Verification items for the finished model (mm, model axes). A direction names the side the tool comes from. Coordinates: 2 decimals unless noted, no trailing zeros. Order: outer loops, then holes, each group sorted by start corner. A loop starts at its lowest first (then second) coordinate and runs counter-clockwise, first axis right, second up. Notation, with made-up numbers: (4, -9.5) -> (26, -9.5) arc R26 cw to (26, 15.5) -> close; hole circle Ø4 at (82.25, -29). An arc over 180 degrees is marked (long way). Use CSV: the item, a comma, the result in double quotes. Start each with the question number.
1) Go/stop test with a flat-tipped pin: pin 1 (2.5 mm diameter, centred on x = -6, z = -2, fed in from +Y). Record where the tip stops, or that it passes through.
2) Scan lines: line 1 along Y through (x, z) = (-5.65, 1.25); line 2 along Z through (x, y) = (-5.75, -19.75); line 3 along Y through (x, z) = (-4.25, -2.3). Record each from-to range of solid material in increasing order.
3) Sectioned sample at C-C on x = -9. Record the boundary of the cut face in (y, z), then the cut area to 3 significant figures.
4) Sectioned sample at D-D on z = 0.35. Record the boundary of the cut face in (x, y).
5) Sectioned sample at B-B on y = -14. Record the boundary of the cut face in (x, z), then the cut area to 3 significant figures.
6) Release check for a two-part mould opening along Y. For faces 1 (the flat face through (-6, -11, 0)), 2 (the flat face through (-6, -23, 0)), 3 (the cylindrical face through (-4.76, -13.44, 1.48)) record: released by +Y, released by -Y, zero draft, split by the parting line, or undercut.
7) Sectioned sample at A-A on x = -5.65. Record the boundary of the cut face in (y, z), then the cut area to 3 significant figures.
8) Tool access check on faces 4 (the flat face through (-6, -13, 3)), 5 (the flat face through (-6, -20, -1)). Record the directions out of +Z, -Z, +X, -X, +Y, -Y that give a thin tool (end or side, any length) a straight path to the whole face; none if there is none.
from build123d import *

# Parameters (mm, degrees)
SKETCH1_W           = 7.7
SKETCH1_H           = 17
SKETCH1_R           = 1.65
BOSS_EXTRUDE1_DEPTH = 3
SKETCH2_W           = 7.7
SKETCH2_H           = 6
BOSS_EXTRUDE2_DEPTH = 3


with BuildPart() as part:
    # Sketch1 → Boss-Extrude1 (new body)
    with BuildSketch(Plane.XY):
        with Locations((-5.65, -11.5)):
            Rectangle(SKETCH1_W, SKETCH1_H)
        with Locations((-5.65, -14.829504021)):
            Circle(SKETCH1_R, mode=Mode.SUBTRACT)
    extrude(amount=BOSS_EXTRUDE1_DEPTH)

    # Sketch2 → Boss-Extrude2 (add)
    with BuildSketch(Plane.XZ.offset(20)):
        with Locations((-5.65, 0)):
            Rectangle(SKETCH2_W, SKETCH2_H)
    extrude(amount=BOSS_EXTRUDE2_DEPTH)


solid = part.part
Answers follow:
1,pin 1,"stops at y = -20"
2,line 1,"y = -23 to -16.48, -13.18 to -3"
2,line 2,"z = 0 to 3"
2,line 3,"y = -23 to -20"
3,outline,"(-23, -3) -> (-20, -3) -> (-20, 0) -> (-3, 0) -> (-3, 3) -> (-23, 3) -> close"
3,area,"69.0 mm²"
4,outline,"(-9.5, -23) -> (-1.8, -23) -> (-1.8, -3) -> (-9.5, -3) -> close; hole circle Ø3.3 at (-5.65, -14.83)"
5,outline,"(-9.5, 0) -> (-7.08, 0) -> (-7.08, 3) -> (-9.5, 3) -> close; (-4.22, 0) -> (-1.8, 0) -> (-1.8, 3) -> (-4.22, 3) -> close"
5,area,"14.5 mm²"
6,face 1,"zero draft"
6,face 2,"released by -Y"
6,face 3,"undercut"
7,outline,"(-23, -3) -> (-20, -3) -> (-20, 0) -> (-16.48, 0) -> (-16.48, 3) -> (-23, 3) -> close; (-13.18, 0) -> (-3, 0) -> (-3, 3) -> (-13.18, 3) -> close"
7,area,"59.1 mm²"
8,face 4,"+Z, +X, -X, +Y, -Y"
8,face 5,"-Z, +X, -X, +Y"
